For this review, take the finished solid that the model builds, in its own axes (mm). Face numbers are marked on the shaded views. A direction names the side the tool comes from. Round coordinates to 2 decimals unless told otherwise and drop trailing zeros. Write each loop counter-clockwise with the first axis right and the second up, starting at its lowest first coordinate (ties: lowest second). Pieces come first, ordered by that corner, then holes.
from build123d import *

# Parameters (mm, degrees)
F0_W     = 55
F0_H     = 21
F1_DEPTH = 2
F2_R     = 1.9
F3_DEPTH = 8
F4_W     = 24.3
F4_H     = 12.3
F5_DEPTH = 8.001


with BuildPart() as f1:
    # F0 (on Front) → F1 (new body)
    with BuildSketch(Plane.XZ):
        with Locations((-0.079613, -4.502098)):
            Rectangle(F0_W, F0_H)
    extrude(amount=F1_DEPTH)

    # F2 (on Front) → F3 (join)
    with BuildSketch(Plane.XZ):
        with Locations((-25.681152, -4.425638)):
            Circle(F2_R)
        with Locations((-17.604692, 3.497164)):
            Circle(F2_R)
        with Locations((-9.68189, -4.579296)):
            Circle(F2_R)
        with Locations((-17.75835, -12.502098)):
            Circle(F2_R)
    extrude(amount=F3_DEPTH)

    # F4 (on Front) → F5 (cut, through all)
    with BuildSketch(Plane.XZ):
        with Locations((9.66811, -4.452098)):
            Rectangle(F4_W, F4_H)
    extrude(amount=F5_DEPTH, mode=Mode.SUBTRACT)


solid = f1.part
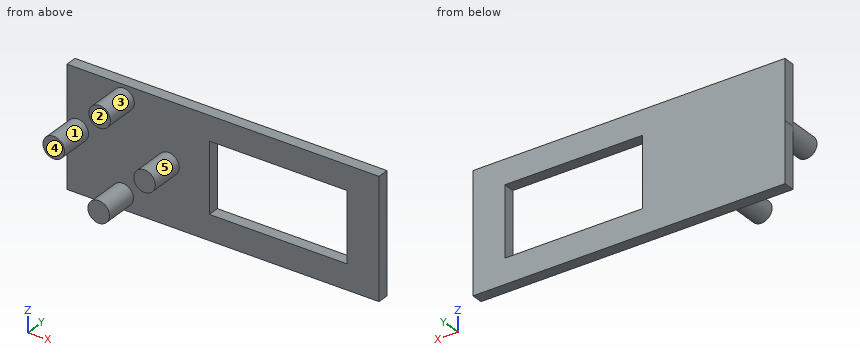
(1) We need section D-D, the plane x = -18.5. Give the boundary of the cut face in (y, z).
Geometry check:
outline: (-8, -14.25) - (-2, -14.25) - (-2, -15) - (0, -15) - (0, 6) - (-2, 6) - (-2, 5.17) - (-8, 5.17) - (-8, 1.82) - (-2, 1.82) - (-2, -10.75) - (-8, -10.75) - close
(2) We need section B-B, the plane x = 0.5. Give the boundary of the cut face in (y, z), and give its area (3 significant figures).
Geometry check:
outline: (-2, -15) - (0, -15) - (0, -10.6) - (-2, -10.6) - close; (-2, 1.7) - (0, 1.7) - (0, 6) - (-2, 6) - close
area: 17.4 mm2
(3) We need section C-C, the plane y = -1.5. Give the boundary of the cut face in (x, z), and give its area (3 significant figures).
Geometry check:
outline: (-27.58, -15) - (27.42, -15) - (27.42, 6) - (-27.58, 6) - (-27.58, -4.35) arc R1.9 ccw to (-27.58, -4.5) - close; hole (-2.48, -10.6) - (21.82, -10.6) - (21.82, 1.7) - (-2.48, 1.7) - close
area: 856 mm2
(4) We need section A-A, the plane z = -9. Give the boundary of the cut face in (x, y).
Geometry check:
outline: (-27.58, -2) - (-2.48, -2) - (-2.48, 0) - (-27.58, 0) - close; (21.82, -2) - (27.42, -2) - (27.42, 0) - (21.82, 0) - close
(5) For pin 1 Ø4 at (x, z) = (21.5, -5) entering from +Y; pin 2 Ø4 at (y, z) = (-6, 2) entering from -X, all flat-tipped, find the tip position at first contact; note any pin that passes through.
Geometry check:
pin 1: stops at y = 0
pin 2: stops at x = -19.5
(6) For line 1 along X through (y, z) = (-1, -9.5); line 2 along Z through (x, y) = (8.5, -0.5); line 3 along Y through (x, z) = (25, -4.75), list the stretches that pass through material, from the lowest coordinate up.
Geometry check:
line 1: x = -27.58 to -2.48, 21.82 to 27.42
line 2: z = -15 to -10.6, 1.7 to 6
line 3: y = -2 to 0
(7) For the marked faces 4 and 5, list the 3-axis set-ups (+Z, -Z, +X, -X, +Y, -Y) from which the entire face can be reached by the end or side of a thin tool; tool diameter is ignored.
Geometry check:
face 4: +Z, -Z, +X, -X, -Y
face 5: -Y
(8) Mouldability with a two-part tool opening along Z and no side actions: class the marked faces 1, 2 and 3 as pulls with the +Z half, pulls with the -Z half, needs draft (parallel to the pull), parting line crosses it, or undercut.
Geometry check:
face 1: parting line crosses it
face 2: needs draft
face 3: undercut
